Part model, mm, in its own coordinate system. Round coordinates to 2 decimals unless told otherwise and drop trailing zeros. Order: outer loops, then holes, each group sorted by start corner. A loop starts at its lowest first (then second) coordinate and runs counter-clockwise, first axis right, second up. Notation, with made-up numbers: (63, 1.5) -> (74, 1.5) arc R23 cw to (74, 34.5) -> close; hole circle Ø5 at (9, 26). An arc over 180 degrees is marked (long way). Return JSON: item names as keys, results as strings. Group by question number.
Autodesk Inventor part; units mm, degrees
ref_plane "YZ Plane" through (0, 0, 0) normal (1, 0, 0) x (0, 1, 0)
ref_plane "XZ Plane" through (0, 0, 0) normal (0, 1, 0) x (-1, 0, 0)
ref_plane "XY Plane" through (0, 0, 0) normal (0, 0, 1) x (1, 0, 0)
sketch "スケッチ1" plane through (0, 0, 0) normal (0, 0, 1) x (1, 0, 0)
  line L0 (0, 0) -> (-4, 0) construction
  circle A0 centre (-4, 0) radius 1.495
  line L1 (0, 0) -> (0, -4) construction
  circle A1 centre (0, -4) radius 1.495
  line L2 (0, 0) -> (4, 0) construction
  circle A2 centre (4, 0) radius 1.495
  line L3 (0, 0) -> (0, 4) construction
  circle A3 centre (0, 4) radius 1.495
  line L4 (0, 0) -> (-8.8388, 8.8388) construction
  circle A4 centre (-8.8388, 8.8388) radius 1.5
  line L5 (0, 0) -> (-8.8388, -8.8388) construction
  circle A5 centre (-8.8388, -8.8388) radius 1.5
  line L6 (0, 0) -> (8.8388, -8.8388) construction
  circle A6 centre (8.8388, -8.8388) radius 1.5
  line L7 (0, 0) -> (8.8388, 8.8388) construction
  circle A7 centre (8.8388, 8.8388) radius 1.5
  circle A8 centre (0, 0) radius 7.295
  circle A9 centre (0, 0) radius 15.5
  circle A10 centre (0, 0) radius 1.995
  dimension "d0" = 4
  dimension "d1" = 2.99
  dimension "d4" = 360
  dimension "d6" = 12.5
  dimension "d7" = 3
  dimension "d8" = 45
  dimension "d11" = 360
  dimension "d13" = 1.8
  dimension "d14" = 14.59
  dimension "d15" = 1.5
  dimension "d16" = 3.99
extrude "押し出し1" add sketch "スケッチ1" along normal blind 4 contours A8
properties part number "脚中間フレームカム" material "アルミニウム 7075"
(1) Saw through at A-A, the plane x = 0. List the corners of the cut face in (y, z) (3 decimals).
(2) Pin check, flat tip, straight feed: P1, Ø1.5, axis at x = -1.5, z = 2.5, coming from the +Y side. Stop position of the tip, or through.
(3) Saw through at D-D, the plane z = 3.2. List the corners of the cut face in (x, y) (3 decimals).
(4) Saw through at C-C, the plane y = -4. List the corners of the cut face in (x, z) (3 decimals).
(5) Probe L1, parallel to Y at x = 0, z = 2.6 (3 decimals); L2, parallel to Y at x = -0.75, z = 1.4; L3, parallel to X at y = 1, z = 0.5. List the from-to ranges inside material, lowest first. Write a range as [from, to].
(6) Mould opens along X. For faces 1 (the cylindrical face through (-1.58, 7.12, 1.97)), 2 (the flat face through (2, -2, 4)), 3 (the cylindrical face through (-2.62, 0.57, 1.97)) say: pulls with the +X half, pulls with the -X half, needs draft (parallel to the pull), parting line crosses it, or undercut.
Results are:
{
 "1": {"outline": "(-7.295, 0) -> (-5.495, 0) -> (-5.495, 4) -> (-7.295, 4) -> close; (-2.505, 0) -> (-1.995, 0) -> (-1.995, 4) -> (-2.505, 4) -> close; (1.995, 0) -> (2.505, 0) -> (2.505, 4) -> (1.995, 4) -> close; (5.495, 0) -> (7.295, 0) -> (7.295, 4) -> (5.495, 4) -> close"},
 "2": {"P1": "stops at y = 7.26"},
 "3": {"outline": "circle Ø14.59 at (0, 0); hole circle Ø2.99 at (-4, 0); hole circle Ø3.99 at (0, 0); hole circle Ø2.99 at (0, -4); hole circle Ø2.99 at (0, 4); hole circle Ø2.99 at (4, 0)"},
 "4": {"outline": "(-6.101, 0) -> (-1.495, 0) -> (-1.495, 4) -> (-6.101, 4) -> close; (1.495, 0) -> (6.101, 0) -> (6.101, 4) -> (1.495, 4) -> close"},
 "5": {"L1": "y = [-7.295, -5.495], [-2.505, -1.995], [1.995, 2.505], [5.495, 7.295]", "L2": "y = [-7.26, -5.29], [-2.71, -1.85], [1.85, 2.71], [5.29, 7.26]", "L3": "x = [-7.23, -5.11], [-2.89, -1.73], [1.73, 2.89], [5.11, 7.23]"},
 "6": {"face 1": "parting line crosses it", "face 2": "needs draft", "face 3": "undercut"}
}
